Geometry: final body of the model. Coordinates: model frame, mm. Face numbers are marked on the shaded views. Give positions to 0.01 mm unless a question says otherwise; leave off trailing zeros. Order: outer loops, then holes, each group sorted by start corner. A loop starts at its lowest first (then second) coordinate and runs counter-clockwise, first axis right, second up. Notation, with made-up numbers: (-18.5, 85) - (18.5, 85) arc R13 cw to (18.5, 100) - close; hole circle Ø8 at (26.25, -18). An arc over 180 degrees is marked (long way). One line per item, written item: value.
```python
from build123d import *

# Parameters (mm, degrees)
SM_BASE_FLANGE_1_DEPTH     = 250
CHAMFER_2_SIZE             = 1
CUT_EXTRUDE_1_DEPTH        = 523.807804073
PATTERN_CIRCULAR_1_COUNT   = 4
PATTERN_CIRCULAR_1_ANGLE   = 90
F_1_THE_OTHER_WAY_COUNT    = 4
F_1_THE_OTHER_WAY_ANGLE    = 90
CHAMFER_1_SIZE             = 3
HOLE_WIZARD_M61_AT_2_COUNT = 2
HOLE_WIZARD_M61_AT_2_PITCH = 136
HOLE_WIZARD_M61_AT_3_COUNT = 2
HOLE_WIZARD_M61_AT_3_PITCH = 272
HOLE_WIZARD_M61_AT_4_COUNT = 2
HOLE_WIZARD_M61_AT_4_PITCH = 408


# Sheet-metal steps are written as plain solids
with BuildPart() as part:
    # Sketch 2 → Базовая кромка1 (new, symmetric)
    with BuildSketch(Plane.XY):
        with BuildLine():
            Line((100, 95), (100, 0))
            ThreePointArc((100, 0), (0, -100), (-100, 0))
            Line((-100, 0), (-100, 95))
            Line((-100, 95), (-108, 95))
            Line((-108, 95), (-108, 0))
            ThreePointArc((-108, 0), (0, -108), (108, 0))
            Line((108, 0), (108, 95))
            Line((108, 95), (100, 95))
        make_face()
    extrude(amount=SM_BASE_FLANGE_1_DEPTH, both=True)

    # Фаска2
    chamfer_2_edges = [part.edges().sort_by_distance(p)[0] for p in [
        (100, 47.5, 250),
        (0, -100, 250),
        (-100, 47.5, 250),
        (0, -100, -250),
        (100, 47.5, -250),
        (-100, 47.5, -250),
    ]]
    chamfer(chamfer_2_edges, length=CHAMFER_2_SIZE)

    # Эскиз7 → Вырез-Вытянуть1 (cut, symmetric)
    with BuildSketch(Plane.XY.offset(250)):
        Polygon((0, 0), (-4, -102.92230079), (4, -102.92230079), align=None)
    cut_extrude_1 = extrude(amount=CUT_EXTRUDE_1_DEPTH, both=True, mode=Mode.SUBTRACT)

    # Круговой массив1: Вырез-Вытянуть1 ×4 about axis
    pattern_circular_1_axis = Axis((0, 0, 0), (0, 0, -1))
    for i in range(1, PATTERN_CIRCULAR_1_COUNT):
        add(cut_extrude_1.rotate(pattern_circular_1_axis, i * PATTERN_CIRCULAR_1_ANGLE / (PATTERN_CIRCULAR_1_COUNT - 1)), mode=Mode.SUBTRACT)

    # 1 the other way: Вырез-Вытянуть1 ×4 about axis
    f_1_the_other_way_axis = Axis((0, 0, 0), (0, 0, 1))
    for i in range(1, F_1_THE_OTHER_WAY_COUNT):
        add(cut_extrude_1.rotate(f_1_the_other_way_axis, i * F_1_THE_OTHER_WAY_ANGLE / (F_1_THE_OTHER_WAY_COUNT - 1)), mode=Mode.SUBTRACT)

    # Фаска1
    chamfer_1_edges = [part.edges().sort_by_distance(p)[0] for p in [
        (100, 95, 0),
        (-100, 95, 0),
    ]]
    chamfer(chamfer_1_edges, length=CHAMFER_1_SIZE)

    # Эскиз9 → Зенковка для винта с полупотайной головкой M61 (revolve, cut)
    with BuildSketch(Plane(origin=(-100, 75, 204), x_dir=(0, 0, -1), z_dir=(0, 1, 0))):
        Polygon((0, 0), (0, 18.982840043), (3.3, 17), (3.3, 3), (6.3, 0), align=None)
    hole_wizard_m61 = revolve(axis=Axis((-93.65, 75, 204), (-1, 0, 0)), mode=Mode.SUBTRACT)

    # Зенковка для винта с полупотайной головкой M61 at 2: Зенковка для винта с полупотайной головкой M61 ×2
    with Locations(*[(0, 0, -i * HOLE_WIZARD_M61_AT_2_PITCH) for i in range(1, HOLE_WIZARD_M61_AT_2_COUNT)]):
        add(hole_wizard_m61, mode=Mode.SUBTRACT)

    # Зенковка для винта с полупотайной головкой M61 at 3: Зенковка для винта с полупотайной головкой M61 ×2
    with Locations(*[(0, 0, -i * HOLE_WIZARD_M61_AT_3_PITCH) for i in range(1, HOLE_WIZARD_M61_AT_3_COUNT)]):
        add(hole_wizard_m61, mode=Mode.SUBTRACT)

    # Зенковка для винта с полупотайной головкой M61 at 4: Зенковка для винта с полупотайной головкой M61 ×2
    with Locations(*[(0, 0, -i * HOLE_WIZARD_M61_AT_4_PITCH) for i in range(1, HOLE_WIZARD_M61_AT_4_COUNT)]):
        add(hole_wizard_m61, mode=Mode.SUBTRACT)

    # Зеркальное отражение1: Зенковка для винта с полупотайной головкой M61 across plane
    add(hole_wizard_m61.mirror(Plane(origin=(0, 0, 0), x_dir=(0, 0, 1), z_dir=(1, 0, 0))), mode=Mode.SUBTRACT)

    # Зеркальное отражение1 copy 1 sketch → Зеркальное отражение1 copy 1 (revolve, cut)
    with BuildSketch(Plane(origin=(100, 75, 68), x_dir=(0, 0, -1), z_dir=(0, 1, 0))):
        Polygon((0, 0), (0, -18.982840043), (3.3, -17), (3.3, -3), (6.3, 0), align=None)
    revolve(axis=Axis((93.65, 75, 68), (-1, 0, 0)), mode=Mode.SUBTRACT)

    # Зеркальное отражение1 copy 2 sketch → Зеркальное отражение1 copy 2 (revolve, cut)
    with BuildSketch(Plane(origin=(100, 75, -68), x_dir=(0, 0, -1), z_dir=(0, 1, 0))):
        Polygon((0, 0), (0, -18.982840043), (3.3, -17), (3.3, -3), (6.3, 0), align=None)
    revolve(axis=Axis((93.65, 75, -68), (-1, 0, 0)), mode=Mode.SUBTRACT)

    # Зеркальное отражение1 copy 3 sketch → Зеркальное отражение1 copy 3 (revolve, cut)
    with BuildSketch(Plane(origin=(100, 75, -204), x_dir=(0, 0, -1), z_dir=(0, 1, 0))):
        Polygon((0, 0), (0, -18.982840043), (3.3, -17), (3.3, -3), (6.3, 0), align=None)
    revolve(axis=Axis((93.65, 75, -204), (-1, 0, 0)), mode=Mode.SUBTRACT)


solid = part.part
```
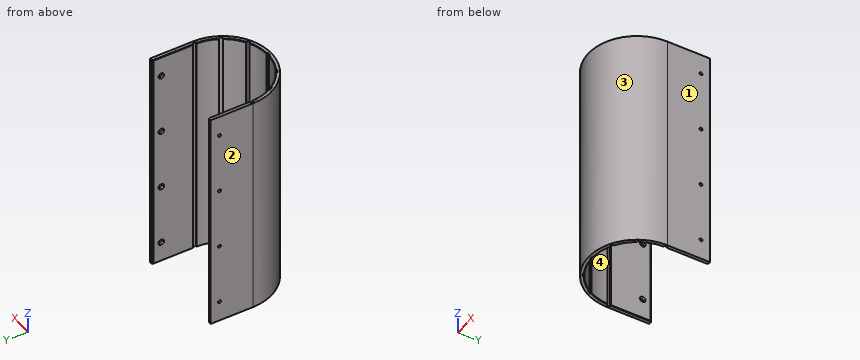
1) Mould query, pull axis X, two halves, no side actions, for the marked faces 1, 2, 3 and 4. Classes: released by +X, released by -X, zero draft, split by the parting line, or undercut.
Answers below:
face 1: released by +X
face 2: released by -X
face 3: split by the parting line
face 4: undercut
2) Section A-A, the plane y = 54. Return loops of the section in (x, z), then the cut area to 3 significant figures.
Answers below:
outline: (-108, -250) - (-101, -250) - (-100, -249) - (-100, 249) - (-101, 250) - (-108, 250) - close; (100, -249) - (101, -250) - (108, -250) - (108, 250) - (101, 250) - (100, 249) - close
area: 8,000 mm^2
3) First-contact query: pin 1 (1 mm diameter, centred on x = -56.5, z = -41, fed in from +Y); pin 2 (2 mm diameter, centred on x = 43.5, z = 175.5, fed in from +Y); pin 3 (4 mm diameter, centred on x = -1.5, z = 97, fed in from +Y); pin 4 (5.5 mm diameter, centred on y = 75, z = -204, fed in from -X) (1 decimal). Flat tips, straight axial feed; report the tip coordinate or a pass-through.
Answers below:
pin 1: y = -82.16
pin 2: y = -89.55
pin 3: y = -102.92
pin 4: through
4) Material intervals for line 1 along Z through (x, y) = (-104.8, 75); line 2 along X through (y, z) = (18, 118); line 3 along X through (y, z) = (-66.5, -5), sorted ascending.
Answers below:
line 1: -250 to -207.3, -200.7 to -71.3, -64.7 to 64.7, 71.3 to 200.7, 207.3 to 250
line 2: -108 to -100, 100 to 108
line 3: -85.1 to -74.68, 74.68 to 85.1
